```python
from build123d import *

# Parameters (mm, degrees)
CROQUIS2_W              = 50
CROQUIS2_H              = 30
SALIENTE_EXTRUIR1_DEPTH = 10
CROQUIS3_R              = 5
CORTAR_EXTRUIR1_DEPTH   = 31.822070015


with BuildPart() as part:
    # Croquis2 → Saliente-Extruir1 (new body)
    with BuildSketch(Plane.YZ):
        Rectangle(CROQUIS2_W, CROQUIS2_H)
    extrude(amount=SALIENTE_EXTRUIR1_DEPTH)

    # Croquis3 → Cortar-Extruir1 (cut, through all)
    with BuildSketch(Plane.YZ.offset(10)):
        with Locations(Location((0, 0, 0), (0, 0, 270))):
            Circle(CROQUIS3_R)
    extrude(amount=-CORTAR_EXTRUIR1_DEPTH, mode=Mode.SUBTRACT)


solid = part.part
```
Here's how the part is built. I have some questions about the finished solid (model axes, mm). Coordinates: 2 decimals unless noted, no trailing zeros. Order: outer loops, then holes, each group sorted by start corner. A loop starts at its lowest first (then second) coordinate and runs counter-clockwise, first axis right, second up. Notation, with made-up numbers: (41, -24) -> (89, -24) arc R21 cw to (89, 8) -> close; hole circle Ø2 at (-20, -13.5). An arc over 180 degrees is marked (long way). Return JSON: item names as keys, results as strings.
1) If I drill on probe 1 along Y at (x, z) = (2.5, 0); probe 2 along Z at (x, y) = (8, -2); probe 3 along Y at (x, z) = (4.5, -1), over which ranges is the centre line in solid material (lowest first)?
Conclusion:
{"probe 1": "y = -25 to -5, 5 to 25", "probe 2": "z = -15 to -4.58, 4.58 to 15", "probe 3": "y = -25 to -4.9, 4.9 to 25"}
2) If we section it at B-B on z = 0: List the corners of the cut face in (x, y) for me, plus the area to 3 significant figures.
Conclusion:
{"outline": "(0, -25) -> (10, -25) -> (10, -5) -> (0, -5) -> close; (0, 5) -> (10, 5) -> (10, 25) -> (0, 25) -> close", "area": "400 mm²"}
3) Thinking about a two-plate mould opening in Y: for faces 1 (the flat face through (5, 0, -15)), 2 (the flat face through (5, 25, 0)), 3 (the flat face through (5, -25, 0)), 4 (the cylindrical face through (5.07, -4.88, 1.08)), which applies, +Y half, -Y half, draft (parallel to the pull), parting line (faces both ways), or undercut?
Conclusion:
{"face 1": "draft", "face 2": "+Y half", "face 3": "-Y half", "face 4": "undercut"}
4) If we section it at A-A on y = 0: List the corners of the cut face in (x, z) for me, plus the area to 3 significant figures.
Conclusion:
{"outline": "(0, -15) -> (10, -15) -> (10, -5) -> (0, -5) -> close; (0, 5) -> (10, 5) -> (10, 15) -> (0, 15) -> close", "area": "200 mm²"}
5) If we section it at C-C on x = 6: List the corners of the cut face in (y, z) for me.
Conclusion:
{"outline": "(-25, -15) -> (25, -15) -> (25, 15) -> (-25, 15) -> close; hole circle Ø10 at (0, 0)"}
6) I'm going to push a flat-ended pin straight in: P1, Ø8, axis at y = -16.5, z = -10.5, coming from the -X side. Where does the tip first touch, or does it pass through?
Conclusion:
{"P1": "stops at x = 0"}
